Can you work these out from the drawing? Everything is in mm from the part's minimum corner. Coordinates: 2 decimals unless noted, no trailing zeros. Loops run counter-clockwise (first coordinate to the right, second up) from the corner with the lowest first, then second, coordinate; pieces in that order, holes last.
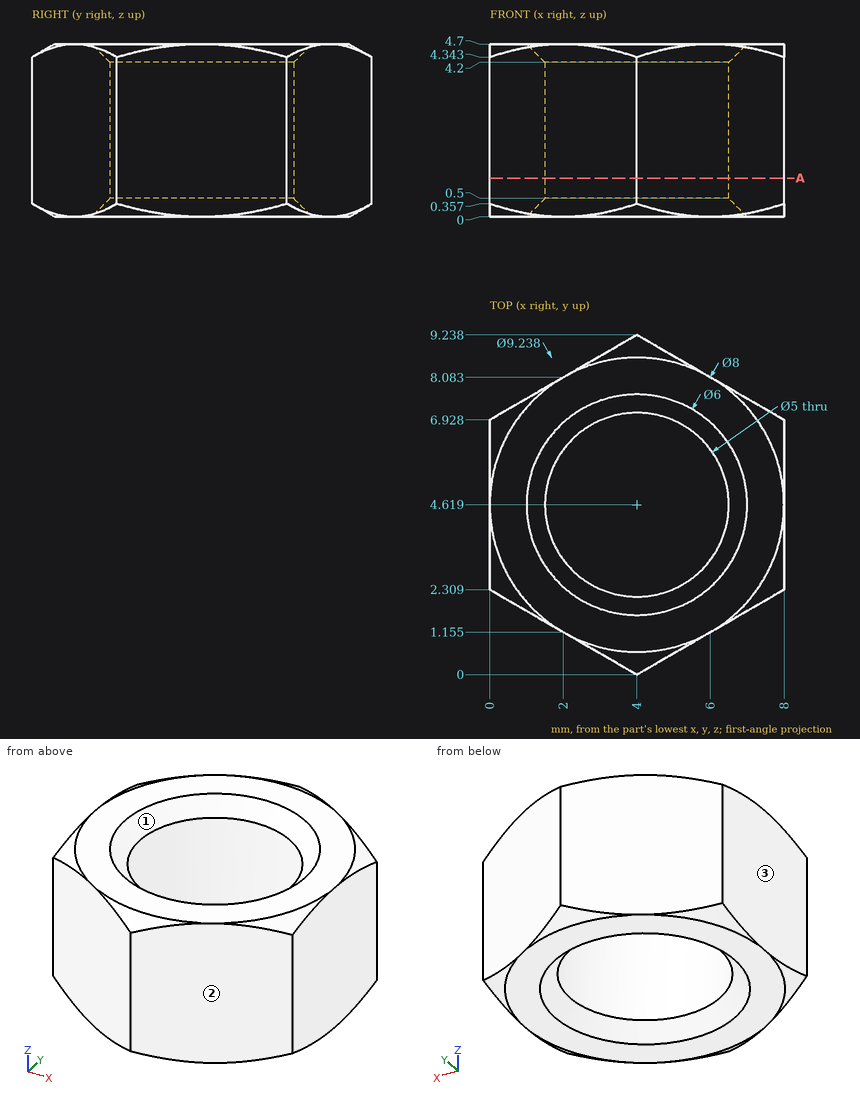
Item 1: I'm going to push flat-ended pins straight in: P1, Ø1.5, axis at x = 2.5, y = 5, coming from the +Z side; P2, Ø1, axis at x = 2, z = 3, coming from the +Y side; P3, Ø1.5, axis at x = 3, z = 1, coming from the +Y side. Where does each tip first touch, or does it pass through?
Results are:
P1: passes through
P2: stops at y = 8.37
P3: stops at y = 9.09
Item 2: I need wall thicknesses on line 1 along X through (y, z) = (5.5, 2.8); line 2 along Y through (x, z) = (5, 1.05); line 3 along Y through (x, z) = (2, 3.85) (1 decimal). Which ranges of each line are inside material? Lowest first, please.
Results are:
line 1: x = 0 to 1.66, 6.34 to 8
line 2: y = 0.58 to 2.33, 6.91 to 8.66
line 3: y = 1.2 to 3.1, 6.1 to 8.1
Item 3: We'd pull the mould along Y, two halves only. Please class the marked faces 1, 2 and 3: +Y half, -Y half, draft (parallel to the pull), parting line (faces both ways), or undercut.
Results are:
face 1: undercut
face 2: -Y half
face 3: draft
Item 4: Suppose I cut it at A-A, the plane z = 1.05. Please give me the cut outline in (x, y), plus the area to 3 significant figures.
Results are:
outline: (0, 2.31) - (4, 0) - (8, 2.31) - (8, 6.93) - (4, 9.24) - (0, 6.93) - close; hole circle Ø5 at (4, 4.62)
area: 35.8 mm2
